from build123d import *

# Parameters (mm, degrees)
SKETCH7_W           = 300
SKETCH7_H           = 100
BOSS_EXTRUDE1_DEPTH = 10
SKETCH1_R           = 2
CUT_EXTRUDE2_DEPTH  = 159.429795178
LPATTERN1_COUNT     = 4
LPATTERN1_PITCH     = 62
SKETCH8_W           = 164.95
SKETCH8_H           = 42
CUT_EXTRUDE3_DEPTH  = 159.429795178
SKETCH10_R          = 2.5
CUT_EXTRUDE4_DEPTH  = 159.429795178


with BuildPart() as part:
    # Sketch7 → Boss-Extrude1 (new body)
    with BuildSketch(Plane.XY):
        Rectangle(SKETCH7_W, SKETCH7_H)
    extrude(amount=-BOSS_EXTRUDE1_DEPTH)

    # Sketch1 → Cut-Extrude2 (cut, through all)
    with BuildSketch(Plane.XY):
        with Locations((4.95, -24.3)):
            Circle(SKETCH1_R)
        with Locations(Location((-4.95, -24.3, 0), (0, 0, 180))):
            Circle(SKETCH1_R)
        with Locations((-4.95, 24.3)):
            Circle(SKETCH1_R)
        with Locations(Location((4.95, 24.3, 0), (0, 0, 180))):
            Circle(SKETCH1_R)
    cut_extrude2 = extrude(amount=-CUT_EXTRUDE2_DEPTH, mode=Mode.SUBTRACT)

    # LPattern1: Cut-Extrude2 ×4
    with Locations(*[(i * LPATTERN1_PITCH, 0, 0) for i in range(1, LPATTERN1_COUNT)]):
        add(cut_extrude2, mode=Mode.SUBTRACT)

    # Sketch8 → Cut-Extrude3 (cut, through all)
    with BuildSketch(Plane.XY):
        with Locations((67.525, 0)):
            Rectangle(SKETCH8_W, SKETCH8_H)
    extrude(amount=-CUT_EXTRUDE3_DEPTH, mode=Mode.SUBTRACT)

    # Sketch10 → Cut-Extrude4 (cut, through all)
    with BuildSketch(Plane.XY):
        with Locations((-120, 20.93113616)):
            Circle(SKETCH10_R)
        with Locations(Location((-120, -20.93113616, 0), (0, 0, 180))):
            Circle(SKETCH10_R)
    extrude(amount=-CUT_EXTRUDE4_DEPTH, mode=Mode.SUBTRACT)


solid = part.part
Here's how the part is built. I have some questions about the finished solid (model axes, mm). A direction names the side the tool comes from. Coordinates: 2 decimals unless noted, no trailing zeros. Write each loop counter-clockwise with the first axis right and the second up, starting at its lowest first coordinate (ties: lowest second). Pieces come first, ordered by that corner, then holes. Notation, with made-up numbers: (-22.5, 15.5) - (-13.5, 15.5) arc R23 cw to (-13.5, 41.5) - close; hole circle Ø6 at (-33, -4). An arc over 180 degrees is marked (long way). Use one line per item in the form item = value.
1) Suppose I cut it at A-A, the plane x = 77. Write out the boundary of the cut face in (y, z).
Solved:
outline = (-50, -10) - (-21, -10) - (-21, 0) - (-50, 0) - close; (21, -10) - (50, -10) - (50, 0) - (21, 0) - close
2) Suppose I cut it at C-C, the plane y = 10.5. Write out the boundary of the cut face in (x, z).
Solved:
outline = (-150, -10) - (-14.95, -10) - (-14.95, 0) - (-150, 0) - close
3) On a 3-axis mill with a long thin cutter (end or side, diameter ignored), from which of +Z, -Z, +X, -X, +Y, -Y can I reach the whole of each face in a straight line? I mean faces 5 (the flat face through (66, 21, -5)), 6 (the flat face through (150, 35, -5)). Say none if no direction works.
Solved:
face_5 = +Z, -Z, +X
face_6 = +Z, -Z, +X, +Y, -Y
4) Thinking about a two-plate mould opening in Y: for faces 1 (the cylindrical face through (-122.385, -21.682, -4.93)), 2 (the flat face through (-2, -50, -5)), 3 (the cylindrical face through (-117.615, 21.682, -4.93)), 4 (the flat face through (-150, -1, -5)), which applies, released by +Y, released by -Y, zero draft, split by the parting line, or undercut?
Solved:
face_1 = undercut
face_2 = released by -Y
face_3 = undercut
face_4 = zero draft
5) Suppose I cut it at B-B, the plane z = -7. Give the number of separate pieces and of enclosed holes in the cut face, plus the area to 3 significant figures.
Solved:
separate_pieces = 1
enclosed_holes = 14
area = 22,900 mm2
6) I'm going to push flat-ended pins straight in: P1, Ø3, axis at x = -4.95, y = 24.3, coming from the +Z side; P2, Ø3, axis at y = -2.5, z = -3, coming from the +X side. Where does each tip first touch, or does it pass through?
Solved:
P1 = through
P2 = -14.95
7) I need wall thicknesses on line 1 (Y direction, x = -4.95, z = -2.5); line 2 (Y direction, x = -120, z = -7); line 3 (Y direction, x = 30, z = -6.5). Which ranges of each line are inside material? Lowest first, please.
Solved:
line_1 = -50 to -26.3, -22.3 to -21, 21 to 22.3, 26.3 to 50
line_2 = -50 to -23.43, -18.43 to 18.43, 23.43 to 50
line_3 = -50 to -21, 21 to 50
